from build123d import *

# Parameters (mm, degrees)
BOSS_EXTRUDE1_DEPTH = 3
SKETCH3_R           = 5.46173703
CUT_EXTRUDE1_DEPTH  = 10
CUT_EXTRUDE2_REACH  = 11.674
SKETCH4_R           = 1.75
SKETCH5_R           = 3
SKETCH5_R_2         = 1.75
BOSS_EXTRUDE2_DEPTH = 5


with BuildPart() as part:
    # Sketch1 → Revolve1 (revolve)
    with BuildSketch(Plane.XY, mode=Mode.PRIVATE) as revolve1_sk:
        Polygon((-0.2, 0), (-0.25, 0), (-4.8, 4.5), (-1.75, 4.5), (-1.75, 2.684678752), align=None)
    revolve(revolve1_sk.sketch.rotate(Axis((0, 0, 0), (0, 1, 0)), 90), axis=Axis((0, 0, 0), (0, 1, 0)))

    # Sketch2 → Boss-Extrude1 (add)
    with BuildSketch(Plane(origin=(0, 4.5, 0), x_dir=(1, 0, 0), z_dir=(0, 1, 0))):
        Polygon((2.309401077, -4), (4.618802154, 0), (2.309401077, 4), (-2.309401077, 4), (-4.618802154, 0), (-2.309401077, -4), align=None)
    extrude(amount=BOSS_EXTRUDE1_DEPTH)

    # Sketch3 → Cut-Extrude1 (cut)
    with BuildSketch(Plane(origin=(0, 7.5, 0), x_dir=(1, 0, 0), z_dir=(0, 1, 0))):
        Circle(SKETCH3_R)
        Polygon((-2.309401077, -4), (2.309401077, -4), (4.618802154, 0), (2.309401077, 4), (-2.309401077, 4), (-4.618802154, 0), align=None, mode=Mode.SUBTRACT)
    extrude(amount=-CUT_EXTRUDE1_DEPTH, mode=Mode.SUBTRACT)

    # Sketch4 → Cut-Extrude2 (cut, up to next)
    with BuildSketch(Plane(origin=(0, 7.5, 0), x_dir=(1, 0, 0), z_dir=(0, 1, 0)), mode=Mode.PRIVATE) as cut_extrude2_sk1:
        with Locations(Location((0, 0, 0), (0, 0, 270))):
            Circle(SKETCH4_R)
    cut_extrude2_tool1 = extrude(cut_extrude2_sk1.sketch, amount=-CUT_EXTRUDE2_REACH, mode=Mode.PRIVATE) & part.part
    add(cut_extrude2_tool1.solids().sort_by_distance((0, 7.5, 0))[0], mode=Mode.SUBTRACT)

    # Sketch5 → Boss-Extrude2 (add)
    with BuildSketch(Plane(origin=(0, 7.5, 0), x_dir=(1, 0, 0), z_dir=(0, 1, 0))):
        with Locations(Location((0, 0, 0), (0, 0, 270))):
            Circle(SKETCH5_R)
        with Locations(Location((0, 0, 0), (0, 0, 270))):
            Circle(SKETCH5_R_2, mode=Mode.SUBTRACT)
    extrude(amount=BOSS_EXTRUDE2_DEPTH)


solid = part.part
Build history of the part. All positions in model axes, mm. A direction names the side the tool comes from. Give positions to 0.01 mm unless a question says otherwise; leave off trailing zeros. Write each loop counter-clockwise with the first axis right and the second up, starting at its lowest first coordinate (ties: lowest second). Pieces come first, ordered by that corner, then holes. Notation, with made-up numbers: (21.5, 71) - (58.5, 71) arc R27 ccw to (58.5, 104) - close; hole circle Ø6 at (3, 11). An arc over 180 degrees is marked (long way). Use one line per item in the form item = value. Start each with the question number.
1. Drop flat-ended pins along their axis: pin 1 Ø4 at (x, z) = (1.5, -2) entering from -Y; pin 2 Ø4 at (y, z) = (5.5, -2.5) entering from -X; pin 3 Ø2 at (x, y) = (-0.5, 11) entering from -Z. Give the stop position or say it passes through.
2. Band-saw the part on A-A on y = 4.75. Write the cut outline in (x, z).
3. 3-axis set-ups, long thin cutter, end or side, ignore diameter. For faces 1 (the face through (-3.448, 5.578, -2.028)), 2 (the face through (3, 7.5, -1)): which of +Z, -Z, +X, -X, +Y, -Y reach the whole face in a straight line?
4. Band-saw the part on B-B on x = 0. Write the cut outline in (y, z).
5. Probe line 1 (X direction, y = 10.6, z = 0); line 2 (Z direction, x = -1, y = 8.75); line 3 (X direction, y = 5.25, z = -0.25). List the from-to ranges inside material, lowest first. Write a range as [from, to].
6. Two-plate mould, pull along Z, no slides. Class faces 3 (the face through (-2, 12.5, 0)), 4 (the face through (3.448, 5.578, 2.028)), 5 (the face through (-0.773, 1.025, -0.172)): released by +Z, released by -Z, zero draft, split by the parting line, or undercut.
7. Band-saw the part on C-C on y = 2.5. Write the cut outline in (x, z), plus the area to 3 significant figures.
Conclusion:
q1.pin_1 = 0.25
q1.pin_2 = -4.33
q1.pin_3 = -3
q2.outline = (-4.62, 0) - (-2.31, -4) - (2.31, -4) - (4.62, 0) - (2.31, 4) - (-2.31, 4) - close; hole circle Ø3.5 at (0, 0)
q3.face_1 = -Z, -X, +Y, -Y
q3.face_2 = +Y
q4.outline = (0, -0.25) - (3.71, -4) - (7.5, -4) - (7.5, -3) - (12.5, -3) - (12.5, -1.75) - (2.68, -1.75) - (0, -0.2) - close; (0, 0.2) - (2.68, 1.75) - (12.5, 1.75) - (12.5, 3) - (7.5, 3) - (7.5, 4) - (3.71, 4) - (0, 0.25) - close
q5.line_1 = [-3, -1.75], [1.75, 3]
q5.line_2 = [-2.83, -1.44], [1.44, 2.83]
q5.line_3 = [-4.47, -1.73], [1.73, 4.47]
q6.face_3 = zero draft
q6.face_4 = released by +Z
q6.face_5 = undercut
q7.outline = circle Ø5.56 at (0, 0); hole circle Ø3.29 at (0, 0)
q7.area = 15.8 mm²
